from build123d import *

# Parameters (mm, degrees)
BOSS_EXTRUDE1_DEPTH = 30
SKETCH2_W           = 1
SKETCH2_H           = 1
SKETCH2_W_2         = 2
SKETCH2_H_2         = 2


with BuildPart() as part:
    # Sketch1 → Boss-Extrude1 (new body)
    with BuildSketch(Plane(origin=(0, 0, 0), x_dir=(0, 0, -1), z_dir=(1, 0, 0))):
        with BuildLine():
            Line((0, 35), (0, 30))
            ThreePointArc((0, 30), (21.213203436, 21.213203436), (30, 0))
            Line((30, 0), (35, 0))
            ThreePointArc((35, 0), (24.748737342, 24.748737342), (0, 35))
        make_face()
    extrude(amount=BOSS_EXTRUDE1_DEPTH)

    # Sketch2 → Cut-Revolve1 (revolve, cut)
    with BuildSketch(Plane.XY):
        with Locations((2.5, 35)):
            Rectangle(SKETCH2_W, SKETCH2_H)
        with Locations((5.5, 35)):
            Rectangle(SKETCH2_W, SKETCH2_H)
        with Locations((8.5, 35)):
            Rectangle(SKETCH2_W, SKETCH2_H)
        with Locations((11.5, 35)):
            Rectangle(SKETCH2_W, SKETCH2_H)
        with Locations((18.5, 35)):
            Rectangle(SKETCH2_W, SKETCH2_H)
        with Locations((21.5, 35)):
            Rectangle(SKETCH2_W, SKETCH2_H)
        with Locations((24.5, 35)):
            Rectangle(SKETCH2_W, SKETCH2_H)
        with Locations((27.5, 35)):
            Rectangle(SKETCH2_W, SKETCH2_H)
        with Locations((15, 34)):
            Rectangle(SKETCH2_W_2, SKETCH2_H_2)
    revolve(axis=Axis((30, 0, 0), (-1, 0, 0)), mode=Mode.SUBTRACT)


solid = part.part
Read the model definition and answer for the solid it produces. Units are mm, in the model's axes. A direction names the side the tool comes from. Coordinates: 2 decimals unless noted, no trailing zeros. Loops run counter-clockwise (first coordinate to the right, second up) from the corner with the lowest first, then second, coordinate; pieces in that order, holes last. Notation, with made-up numbers: (81, -4.5) - (105, -4.5) arc R19 cw to (105, 3.5) - close; hole circle Ø9 at (89.25, 73). An arc over 180 degrees is marked (long way). Answer in a Markdown table with one row per item.
Q1. For faces 3 (the cylindrical face through (0.986, 24.475, -25.019)), 4 (the flat face through (12, 25, -24)), determine the directions among +Z, -Z, +X, -X, +Y, -Y from which every point of the face is accessible in a straight line to the end or side of a thin tool.
Here are the results:
| item | result |
|---|---|
| face 3 | -Z, +X, -X, +Y |
| face 4 | -Z, +Y |
Q2. The mould has two halves that part along X. Classify faces 1 (the cylindrical face through (2.51, 24.66, -24.13)), 2 (the cylindrical face through (9.986, 24.475, -25.019)): pulls with the +X half, pulls with the -X half, needs draft (parallel to the pull), parting line crosses it, or undercut.
Here are the results:
| item | result |
|---|---|
| face 1 | undercut |
| face 2 | needs draft |
Q3. Find section A-A on x = 13.25. Write down the section's boundary in (y, z).
Here are the results:
| item | result |
|---|---|
| outline | (0, -35) arc R35 ccw to (35, 0) - (30, 0) arc R30 cw to (0, -30) - close |
Q4. Straight lines are drawn through the part: line 1 along Z through (x, y) = (17.75, 19); line 2 along Z through (x, y) = (23.5, 10); line 3 along Y through (x, z) = (9.25, -17). For each, find the intervals that lie inside material, in ascending order. Write a range as [from, to].
Here are the results:
| item | result |
|---|---|
| line 1 | z = [-29.39, -23.22] |
| line 2 | z = [-33.54, -28.28] |
| line 3 | y = [24.72, 30.59] |
Q5. Given P1, Ø8, axis at x = 21.5, z = -8.5, coming from the -Y side; P2, Ø1.5, axis at x = 25.5, y = 6.5, coming from the -Z side; P3, Ø1, axis at x = 19.5, y = 29.5, coming from the -Z side, each flat-ended and moving along its own axis, determine where each tip first touches the part or whether it passes through.
Here are the results:
| item | result |
|---|---|
| P1 | stops at y = 27.27 |
| P2 | stops at z = -34.52 |
| P3 | stops at z = -19.6 |
